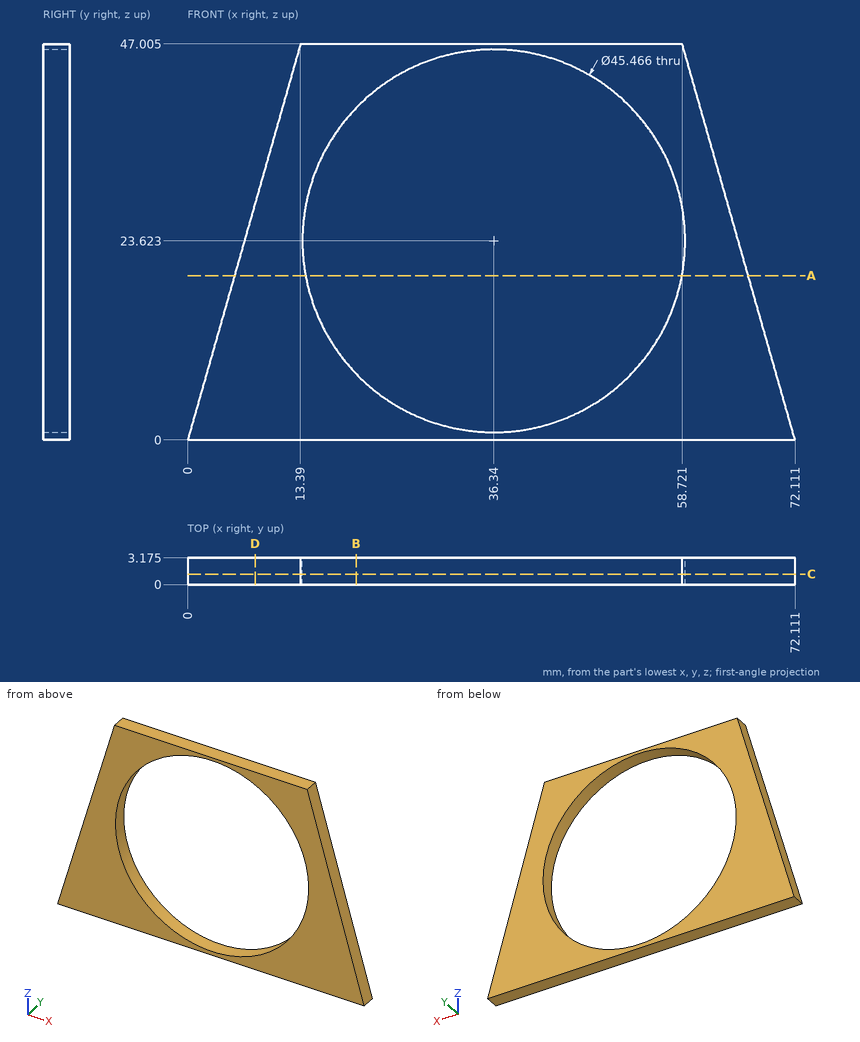
For this review, use the dimensioned drawing (mm, ordinates from the lowest corner) and the shaded views. Give positions to 0.01 mm unless a question says otherwise; leave off trailing zeros. Write each loop counter-clockwise with the first axis right and the second up, starting at its lowest first coordinate (ties: lowest second). Pieces come first, ordered by that corner, then holes.
(1) Consider section D-D, the plane x = 8. Give the boundary of the cut face in (y, z) (1 decimal).
(2) Consider section A-A, the plane z = 19.5. Give the boundary of the cut face in (x, y) (1 decimal).
(3) Consider section B-B, the plane x = 20. Give the boundary of the cut face in (y, z) (1 decimal).
(4) To check wall thickness, follow L1, parallel to Z at x = 37, y = 2.1 (1 decimal); L2, parallel to X at y = 2.55, z = 19; L3, parallel to Z at x = 29.5, y = 0.7 (1 decimal). State the ranges of each line that lie inside material, in increasing order.
(5) Consider section C-C, the plane y = 1.25. Give the boundary of the cut face in (x, z) (1 decimal), and give its area (3 significant figures).
Returned:
1. outline: (0, 0) - (3.2, 0) - (3.2, 28.1) - (0, 28.1) - close
2. outline: (5.6, 0) - (14, 0) - (14, 3.2) - (5.6, 3.2) - close; (58.7, 0) - (66.6, 0) - (66.6, 3.2) - (58.7, 3.2) - close
3. outline: (0, 0) - (3.2, 0) - (3.2, 7.8) - (0, 7.8) - close; (0, 39.4) - (3.2, 39.4) - (3.2, 47) - (0, 47) - close
4. L1: z = 0 to 0.9, 46.3 to 47
4. L2: x = 5.41 to 14.08, 58.6 to 66.7
4. L3: z = 0 to 1.9, 45.3 to 47
5. outline: (0, 0) - (72.1, 0) - (58.7, 47) - (13.4, 47) - close; hole circle Ø45.5 at (36.3, 23.6)
5. area: 1,140 mm2
